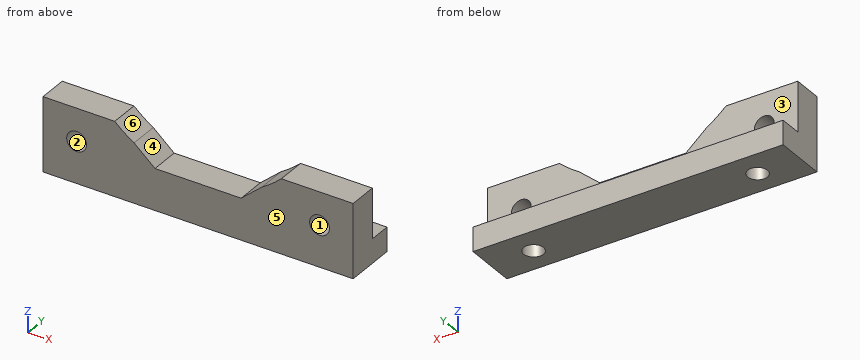
```python
from build123d import *

# Parameters (mm, degrees)
F1_DEPTH = 90
F3_D     = 11.5
F3_DEPTH = 15
F3_TIP   = 3.4549485594
F5_DEPTH = 30.001
F7_D     = 11.5
F9_DEPTH = 30.001


with BuildPart() as f1:
    # F0 (on Right) → F1 (new body, symmetric)
    with BuildSketch(Plane.YZ):
        Polygon((0, 43), (0, 0), (30, 0), (30, 14), (17, 14), (17, 43), align=None)
    extrude(amount=F1_DEPTH, both=True)

    # F3
    with Locations(Plane(origin=(0, 0, 0), x_dir=(1, 0, 0), z_dir=(0, 0, -1))):
        with Locations((65, -14.5), (-65, -14.5)):
            Hole(F3_D / 2, depth=F3_DEPTH)
            with Locations((0, 0, -(F3_DEPTH + F3_TIP / 2))):  # 118° drill point
                Cone(0, F3_D / 2, F3_TIP, mode=Mode.SUBTRACT)

    # F4 (on face) → F5 (cut, through all)
    with BuildSketch(Plane.XZ):
        with BuildLine():
            Line((48.3425278611, 43), (-48.3425278611, 43))
            ThreePointArc((-48.3425278611, 43), (0, 24), (48.3425278611, 43))
        make_face()
    extrude(amount=-F5_DEPTH, mode=Mode.SUBTRACT)

    # F7 (through all)
    with Locations(Plane.XZ):
        with Locations((-70.5, 24), (70.5, 24)):
            Hole(F7_D / 2)

    # F8 (on face) → F9 (cut, through all)
    with BuildSketch(Plane.XZ):
        with BuildLine():
            Line((0, 43), (-47, 43))
            Line((-47, 43), (-37.1565411971, 34.4988310339))
            ThreePointArc((-37.1565411971, 34.4988310339), (-19.305659836, 26.6751033788), (0, 24))
            Line((0, 24), (0, 43))
        make_face()
        with BuildLine():
            ThreePointArc((0, 24), (-19.305659836, 26.6751033788), (-37.1565411971, 34.4988310339))
            Line((-37.1565411971, 34.4988310339), (-25, 24))
            Line((-25, 24), (0, 24))
        make_face()
        with BuildLine():
            Line((47, 43), (0, 43))
            Line((0, 43), (0, 24))
            ThreePointArc((0, 24), (19.305659836, 26.6751033788), (37.1565411971, 34.4988310339))
            Line((37.1565411971, 34.4988310339), (47, 43))
        make_face()
        with BuildLine():
            ThreePointArc((37.1565411971, 34.4988310339), (19.305659836, 26.6751033788), (0, 24))
            Line((0, 24), (25, 24))
            Line((25, 24), (37.1565411971, 34.4988310339))
        make_face()
    extrude(amount=-F9_DEPTH, mode=Mode.SUBTRACT)


solid = f1.part
```
The listing builds one solid part. Answer for the finished solid, in the listing's coordinates (mm). Face numbers are marked on the shaded views. A direction names the side the tool comes from. Round coordinates to 2 decimals unless told otherwise and drop trailing zeros. Order: outer loops, then holes, each group sorted by start corner. A loop starts at its lowest first (then second) coordinate and runs counter-clockwise, first axis right, second up. Notation, with made-up numbers: (-1, 5.25) -> (26, 5.25) arc R20 ccw to (26, 23.25) -> close; hole circle Ø11 at (14.5, -22). An arc over 180 degrees is marked (long way). Answer as CSV lines item,"result". Start each with the question number.
(1) Find the intervals of material crossed by probe 1 along Y at (x, z) = (-65, 11); probe 2 along X at (y, z) = (11.25, 26.5); probe 3 along X at (y, z) = (5, 27), in increasing order. Write a range as from..to.
(2) Flat-ended cylindrical pins translate along their axes: pin 1 Ø4 at (x, y) = (38, 25.5) entering from +Z; pin 2 Ø5 at (x, z) = (-48, 21) entering from +Y; pin 3 Ø5 at (x, y) = (-1, 8) entering from +Z. Find the tip coordinate at first contact, or state that the pin passes through.
(3) A tool of negligible diameter and unlimited length cuts with its end or side. For the marked faces 5 and 6, from which of +Z, -Z, +X, -X, +Y, -Y can it reach the whole face along a straight path? Write none if from no direction.
(4) The part is cut by section A-A (z = 10.5). Determine the outline of the cut face in (x, y), then the cut area to 3 significant figures.
(5) The part is cut by section B-B (x = -21.5). Determine the outline of the cut face in (y, z), then the cut area to 3 significant figures.
(6) The part is cut by section D-D (y = 11.5). Count the separate pieces of the cut face and the enclosed holes in it, then the cut area to 3 significant figures.
(7) The part is cut by section C-C (y = 23.75). Determine the outline of the cut face in (x, z).
(8) For a pull along Z with two mould halves and no side action, classify the marked faces 1, 2, 3 and 4 as +Z half, -Z half, draft (parallel to the pull), parting line (faces both ways), or undercut.
Evaluation:
1,probe 1,"0..8.75, 20.25..30"
1,probe 2,"-90..-75.68, -65.32..-27.89, 27.89..65.32, 75.68..90"
1,probe 3,"-90..-75.41, -65.59..-28.47, 28.47..65.59, 75.41..90"
2,pin 1,"z = 14"
2,pin 2,"y = 17"
2,pin 3,"z = 24"
3,face 5,"+Z, -Z, +X, -X, -Y"
3,face 6,"+Z, +Y, -Y"
4,outline,"(-90, 0) -> (90, 0) -> (90, 30) -> (-90, 30) -> close; hole circle Ø11.5 at (-65, 14.5); hole circle Ø11.5 at (65, 14.5)"
4,area,"5,190 mm²"
5,outline,"(0, 0) -> (30, 0) -> (30, 14) -> (17, 14) -> (17, 24) -> (0, 24) -> close"
5,area,"590 mm²"
6,separate pieces,"1"
6,enclosed holes,"2"
6,area,"5,830 mm²"
7,outline,"(-90, 0) -> (90, 0) -> (90, 14) -> (-90, 14) -> close"
8,face 1,"undercut"
8,face 2,"undercut"
8,face 3,"draft"
8,face 4,"+Z half"
